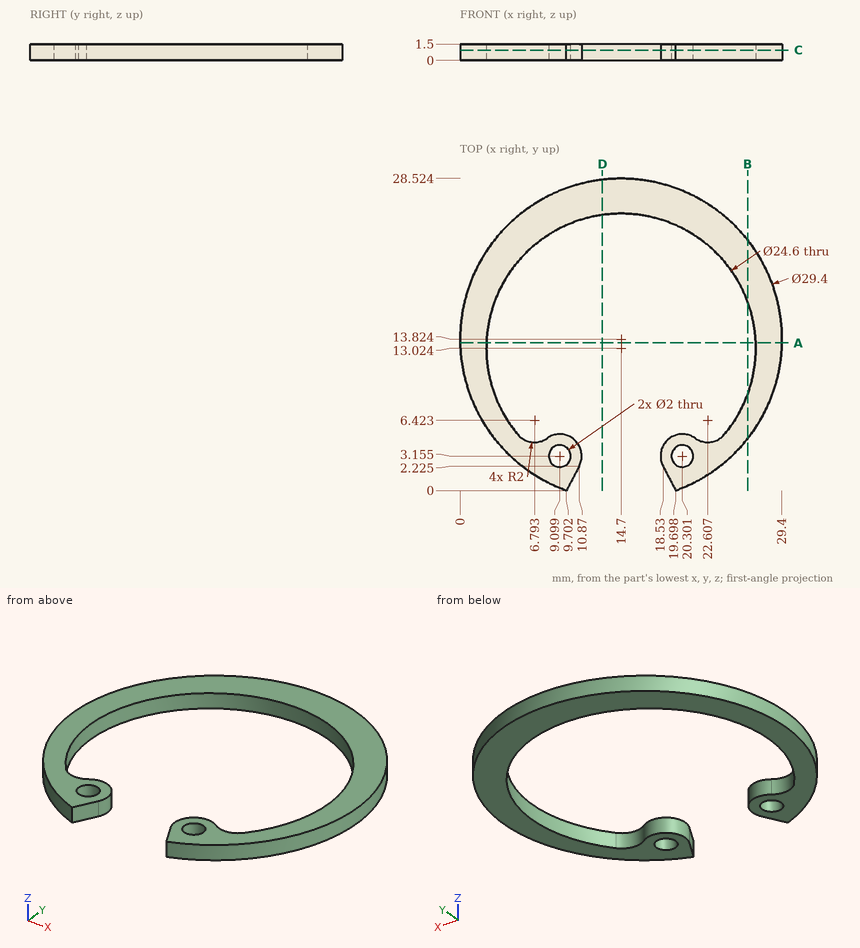
Print and shaded views of the part. All mm, measured from the part's lowest x, y and z. Round coordinates to 2 decimals unless told otherwise and drop trailing zeros. Order: outer loops, then holes, each group sorted by start corner. A loop starts at its lowest first (then second) coordinate and runs counter-clockwise, first axis right, second up.
Q1. Slice it at D-D (x = 13). Write the cut outline in (y, z) (1 decimal).
Q2. Drop a flat-ended pin along its axis: pin 1 (2.5 mm diameter, centred on x = 20.3, y = 3.16, fed in from +Z). Give the stop position or say it passes through.
Q3. Wall check: L1, parallel to Y at x = 23, z = 0.1 (1 decimal); L2, parallel to Y at x = 4.25, z = 0.5 (1 decimal); L3, parallel to X at y = 17.75, z = 0.9 (1 decimal). Give the ranges that are in metal, low to high.
Q4. Slice it at A-A (y = 13.5). Write the cut outline in (x, z).
Q5. Slice it at B-B (x = 26.25). Write the cut outline in (y, z) (1 decimal), and give its area (3 significant figures).
Q6. Slice it at C-C (z = 0.95). Write the cut outline in (x, y) (1 decimal), and give its area (3 significant figures).
Results below:
1. outline: (25.2, 0) - (28.4, 0) - (28.4, 1.5) - (25.2, 1.5) - close
2. pin 1: stops at z = 1.5
3. L1: y = 1.7 to 4.5, 22.1 to 26
3. L2: y = 3.5 to 6.5, 19.5 to 24.2
3. L3: x = 0.5 to 3.3, 26.1 to 28.9
4. outline: (0, 0) - (2.41, 0) - (2.41, 1.5) - (0, 1.5) - close; (26.99, 0) - (29.4, 0) - (29.4, 1.5) - (26.99, 1.5) - close
5. outline: (4.7, 0) - (8.8, 0) - (8.8, 1.5) - (4.7, 1.5) - close; (17.3, 0) - (22.9, 0) - (22.9, 1.5) - (17.3, 1.5) - close
5. area: 14.6 mm2
6. outline: (5.3, 5.1) arc R12.3 cw (long way) to (24.1, 5.1) arc R2 cw to (21.5, 4.8) arc R2 ccw to (18.5, 2.2) - (19.7, 0) arc R14.7 ccw (long way) to (9.7, 0) - (10.9, 2.2) arc R2 ccw to (7.9, 4.8) arc R2 cw to start; hole circle Ø2 at (9.1, 3.2); hole circle Ø2 at (20.3, 3.2)
6. area: 204 mm2
